from build123d import *

# Parameters (mm, degrees)
SKETCH2_R           = 38.1
BOSS_EXTRUDE5_DEPTH = 3.0988
SKETCH2_3_R         = 1.0795
CUT_EXTRUDE3_DEPTH  = 54.970571254


with BuildPart() as part:
    # Sketch2 → Boss-Extrude5 (new body)
    with BuildSketch(Plane(origin=(0, 0, 0), x_dir=(0, 0, -1), z_dir=(1, 0, 0))):
        Circle(SKETCH2_R)
    extrude(amount=BOSS_EXTRUDE5_DEPTH)

    # Sketch2_3 → Cut-Extrude3 (cut, through all)
    with BuildSketch(Plane(origin=(0, 0, 0), x_dir=(0, 0, -1), z_dir=(1, 0, 0))):
        with BuildLine():
            Line((21.253442374, -18.136559411), (0, -5.865878735))
            Line((0, -5.865878735), (-21.253442374, -18.136559411))
            ThreePointArc((-21.253442374, -18.136559411), (0, -27.94), (21.253442374, -18.136559411))
        make_face()
        with BuildLine():
            Line((-26.333442374, -9.337741308), (-5.08, 2.932939367))
            Line((-5.08, 2.932939367), (-5.08, 27.474300719))
            ThreePointArc((-5.08, 27.474300719), (-24.196749782, 13.97), (-26.333442374, -9.337741308))
        make_face()
        with BuildLine():
            Line((5.08, 2.932939367), (26.333442374, -9.337741308))
            ThreePointArc((26.333442374, -9.337741308), (27.535431538, -4.737468737), (27.94, 0))
            ThreePointArc((27.94, 0), (21.477648847, 17.870484045), (5.08, 27.474300719))
            Line((5.08, 27.474300719), (5.08, 2.932939367))
        make_face()
        Circle(SKETCH2_3_R)
    extrude(amount=CUT_EXTRUDE3_DEPTH, mode=Mode.SUBTRACT)


solid = part.part
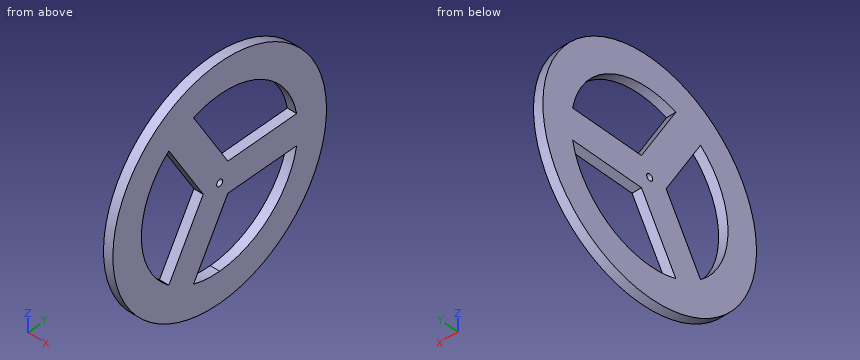
The listing builds one solid part. Answer for the finished solid, in the listing's coordinates (mm). Round coordinates to 2 decimals unless told otherwise and drop trailing zeros. Write each loop counter-clockwise with the first axis right and the second up, starting at its lowest first coordinate (ties: lowest second). Pieces come first, ordered by that corner, then holes. Notation, with made-up numbers: (49, 72.25) - (89, 72.25) arc R19 cw to (89, 105.25) - close; hole circle Ø4 at (54.25, 53.5). An arc over 180 degrees is marked (long way). Use one line per item in the form item = value. Start each with the question number.
Item 1: A cutting plane is placed at B-B (y = -14.5). Write down the section's boundary in (x, z), plus the area to 3 significant figures.
Item 2: A cutting plane is placed at D-D (y = -3.5). Write down the section's boundary in (x, z), plus the area to 3 significant figures.
Item 3: A cutting plane is placed at C-C (z = 12.5). Write down the section's boundary in (x, y), plus the area to 3 significant figures.
Item 4: Find the intervals of material crossed by line 1 (Y direction, x = 2.4, z = 0); line 2 (Y direction, x = 1.95, z = 8); line 3 (Y direction, x = 1.2, z = -4.5), in increasing order. Write a range as [from, to].
Item 5: A cutting plane is placed at A-A (x = 2.5). Write down the section's boundary in (y, z), plus the area to 3 significant figures.
Item 6: Flat-ended cylindrical pins translate along their axes: pin 1 Ø1 at (x, z) = (0.5, -18.5) entering from -Y; pin 2 Ø1.5 at (x, y) = (2, 16.5) entering from -Z; pin 3 Ø1 at (x, z) = (2.5, -11) entering from +Y. Find the tip coordinate at first contact, or state that the pin passes through.
The answers:
q1.outline = (0, -35.23) - (3.1, -35.23) - (3.1, -14.95) - (0, -14.95) - close; (0, 14.95) - (3.1, 14.95) - (3.1, 35.23) - (0, 35.23) - close
q1.area = 126 mm^2
q2.outline = (0, -37.94) - (3.1, -37.94) - (3.1, -27.72) - (0, -27.72) - close; (0, -16.22) - (3.1, -16.22) - (3.1, 16.22) - (0, 16.22) - close; (0, 27.72) - (3.1, 27.72) - (3.1, 37.94) - (0, 37.94) - close
q2.area = 164 mm^2
q3.outline = (0, -35.99) - (3.1, -35.99) - (3.1, -24.99) - (0, -24.99) - close; (0, -13.08) - (3.1, -13.08) - (3.1, -1.35) - (0, -1.35) - close; (0, 24.99) - (3.1, 24.99) - (3.1, 35.99) - (0, 35.99) - close
q3.area = 105 mm^2
q4.line_1 = [-38.1, -27.94], [-5.87, -1.08], [1.08, 38.1]
q4.line_2 = [-37.25, -26.77], [-10.48, 1.25], [26.77, 37.25]
q4.line_3 = [-37.83, -27.58], [-8.46, 37.83]
q5.outline = circle Ø76.2 at (0, 0); hole (-18.14, -21.25) - (-5.87, 0) - (-18.14, 21.25) arc R27.94 ccw to start; hole (-9.34, -26.33) arc R27.94 ccw to (27.47, -5.08) - (2.93, -5.08) - close; hole (-9.34, 26.33) - (2.93, 5.08) - (27.47, 5.08) arc R27.94 ccw to start; hole circle Ø2.16 at (0, 0)
q5.area = 2,910 mm^2
q6.pin_1 = -33.58
q6.pin_2 = -34.69
q6.pin_3 = 36.62
